Check sheet for the modelled part. Datum: model origin and axes. Units: mm. A direction names the side the tool comes from. Round coordinates to 2 decimals unless told otherwise and drop trailing zeros. Write each loop counter-clockwise with the first axis right and the second up, starting at its lowest first coordinate (ties: lowest second). Pieces come first, ordered by that corner, then holes. Notation, with made-up numbers: (47.5, 41.5) -> (63.5, 41.5) arc R4 cw to (63.5, 46.5) -> close; hole circle Ø2 at (43, -22.75). An arc over 180 degrees is marked (long way). One line per item, written item: value.
from build123d import *

# Parameters (mm, degrees)
SKETCH1_W                                = 95
SKETCH1_H                                = 54
BOSS_EXTRUDE1_DEPTH                      = 10
SKETCH2_W                                = 95
SKETCH2_H                                = 54
SKETCH2_W_2                              = 93
SKETCH2_H_2                              = 52
CUT_EXTRUDE1_DEPTH                       = 1
CBORE_FOR_M3_PAN_HEAD_SCREW1_D           = 3.4
CBORE_FOR_M3_PAN_HEAD_SCREW1_CBORE_D     = 7
CBORE_FOR_M3_PAN_HEAD_SCREW1_CBORE_DEPTH = 2.4
CHAMFER1_SIZE                            = 1
SKETCH4_R                                = 8
CUT_EXTRUDE2_DEPTH                       = 10


with BuildPart() as part:
    # Sketch1 → Boss-Extrude1 (new body)
    with BuildSketch(Plane.XY):
        with Locations((-407.351708977, 0)):
            Rectangle(SKETCH1_W, SKETCH1_H)
    extrude(amount=BOSS_EXTRUDE1_DEPTH)

    # Sketch2 → Cut-Extrude1 (cut)
    with BuildSketch(Plane.XY.offset(10)):
        with Locations((-407.351708977, 0)):
            Rectangle(SKETCH2_W, SKETCH2_H)
        with Locations((-407.351708977, 0)):
            Rectangle(SKETCH2_W_2, SKETCH2_H_2, mode=Mode.SUBTRACT)
    extrude(amount=-CUT_EXTRUDE1_DEPTH, mode=Mode.SUBTRACT)

    # CBORE for M3 Pan Head Screw1 (through all)
    with Locations(Plane(origin=(-448.851708977, 21, 10), x_dir=(1, 0, 0), z_dir=(0, 0, 1))):
        with Locations((0, 0), (83, 0), (83, -42), (0, -42)):
            CounterBoreHole(CBORE_FOR_M3_PAN_HEAD_SCREW1_D / 2, CBORE_FOR_M3_PAN_HEAD_SCREW1_CBORE_D / 2, CBORE_FOR_M3_PAN_HEAD_SCREW1_CBORE_DEPTH)

    # Chamfer1
    chamfer1_edges = [part.edges().sort_by_distance(p)[0] for p in [
        (-452.351708977, -21, 10),
        (-369.351708977, -21, 10),
        (-369.351708977, 21, 10),
        (-452.351708977, 21, 10),
    ]]
    chamfer(chamfer1_edges, length=CHAMFER1_SIZE)

    # Sketch4 → Cut-Extrude2 (cut)
    with BuildSketch(Plane.XY.offset(10)):
        with Locations((-407.351708977, 15)):
            Circle(SKETCH4_R)
        with Locations((-407.351708977, -15)):
            Circle(SKETCH4_R)
    extrude(amount=-CUT_EXTRUDE2_DEPTH, mode=Mode.SUBTRACT)


solid = part.part
Item 1: Sectioned sample at B-B (z = 2.25). Enter the section's corners in (x, y), then the cut area to 3 significant figures.
Result set:
outline: (-454.85, -27) -> (-359.85, -27) -> (-359.85, 27) -> (-454.85, 27) -> close; hole circle Ø3.4 at (-448.85, -21); hole circle Ø3.4 at (-448.85, 21); hole circle Ø16 at (-407.35, -15); hole circle Ø16 at (-407.35, 15); hole circle Ø3.4 at (-365.85, -21); hole circle Ø3.4 at (-365.85, 21)
area: 4,690 mm^2
Item 2: Material ranges on line 1 along Y through (x, z) = (-366, 4.5); line 2 along Y through (x, z) = (-413.5, 7); line 3 along X through (y, z) = (-18.5, 8.75), recorded low to high.
Result set:
line 1: -27 to -22.69, -19.31 to 19.31, 22.69 to 27
line 2: -27 to -20.12, -9.88 to 9.88, 20.12 to 27
line 3: -454.85 to -451.3, -446.4 to -414.55, -400.16 to -368.3, -363.4 to -359.85
Item 3: Release check for a two-part mould opening along X. For faces 3 (the flat face through (-408, -27, 4)), 4 (the cylindrical face through (-362.513, -19.949, 8.31)) record: pulls with the +X half, pulls with the -X half, needs draft (parallel to the pull), parting line crosses it, or undercut.
Result set:
face 3: needs draft
face 4: undercut
Item 4: Sectioned sample at D-D (y = 8). Enter the section's corners in (x, z), then the cut area to 3 significant figures.
Result set:
outline: (-454.85, 0) -> (-411.22, 0) -> (-411.22, 10) -> (-453.85, 10) -> (-453.85, 9) -> (-454.85, 9) -> close; (-403.48, 0) -> (-359.85, 0) -> (-359.85, 9) -> (-360.85, 9) -> (-360.85, 10) -> (-403.48, 10) -> close
area: 871 mm^2
Item 5: Sectioned sample at C-C (y = -21). State how many separate pieces and enclosed holes the cut face has, then the cut area to 3 significant figures.
Result set:
separate pieces: 4
enclosed holes: 0
area: 755 mm^2
Item 6: Sectioned sample at A-A (y = -15). Enter the section's corners in (x, z), then the cut area to 3 significant figures.
Result set:
outline: (-454.85, 0) -> (-415.35, 0) -> (-415.35, 10) -> (-453.85, 10) -> (-453.85, 9) -> (-454.85, 9) -> close; (-399.35, 0) -> (-359.85, 0) -> (-359.85, 9) -> (-360.85, 9) -> (-360.85, 10) -> (-399.35, 10) -> close
area: 788 mm^2
Item 7: Depth check by flat-ended pin: pin 1 (0.5 mm diameter, centred on x = -391.5, z = 9.5, fed in from +Y); pin 2 (3.5 mm diameter, centred on x = -447.5, y = -21, fed in from +Z); pin 3 (2.5 mm diameter, centred on x = -365.85, y = 21, fed in from +Z); pin 4 (0.5 mm diameter, centred on y = -8.5, z = 9.5, fed in from +X). Enter the tip coordinate at first touch or a pass-through.
Result set:
pin 1: y = 26
pin 2: z = 7.6
pin 3: through
pin 4: x = -360.85
Item 8: Tool access check on faces 1 (the cylindrical face through (-450.473, 21.511, 3.747)), 2 (the cylindrical face through (-445.513, -19.949, 8.31)). Record the directions out of +Z, -Z, +X, -X, +Y, -Y that give a thin tool (end or side, any length) a straight path to the whole face; none if there is none.
Result set:
face 1: +Z, -Z
face 2: +Z
